Input: dimensioned drawing with shaded views. Units: mm. Origin: part minimum x, y, z. A direction names the side the tool comes from. Round coordinates to 2 decimals unless told otherwise and drop trailing zeros. Order: outer loops, then holes, each group sorted by start corner. A loop starts at its lowest first (then second) coordinate and runs counter-clockwise, first axis right, second up. Notation, with made-up numbers: M 67,60.5 L 122,60.5 A27 ccw 122,82.5 Z; hole C 88,72 d11. An arc over 180 degrees is marked long. Put each result on its own line as item: value. Start each with the question number.
1) Material intervals for probe 1 along Z at (x, y) = (110, 31); probe 2 along X at (y, z) = (25.5, 97.5); probe 3 along Z at (x, y) = (126, 18), sorted ascending. Write a range as [from, to].
2) Section A-A, the plane x = 110. Count the separate pieces of the cut face and the enclosed holes in it, then the cut area to 3 significant figures.
3) First-contact query: P1, Ø10.5, axis at x = 75.5, z = 110, coming from the +Y side; P2, Ø1, axis at y = 14, z = 62.5, coming from the +X side; P3, Ø3, axis at y = 49.5, z = 53, coming from the +X side. Flat tips, straight axial feed; report the tip coordinate or a pass-through.
4) Draft query along Z for the marked faces 1, 2 and 3. Return one class per face: pulls with the +Z half, pulls with the -Z half, needs draft (parallel to the pull), parting line crosses it, or undercut.
5) Section C-C, the plane y = 48. Return loops of the section in (x, z).
6) Access query for the marked faces 4, 5 and 6. Directions: +Z, -Z, +X, -X, +Y, -Y. A direction counts if a zero-diameter tool reaches every point of the face in a straight line with its end or side. Return the directions, or none.
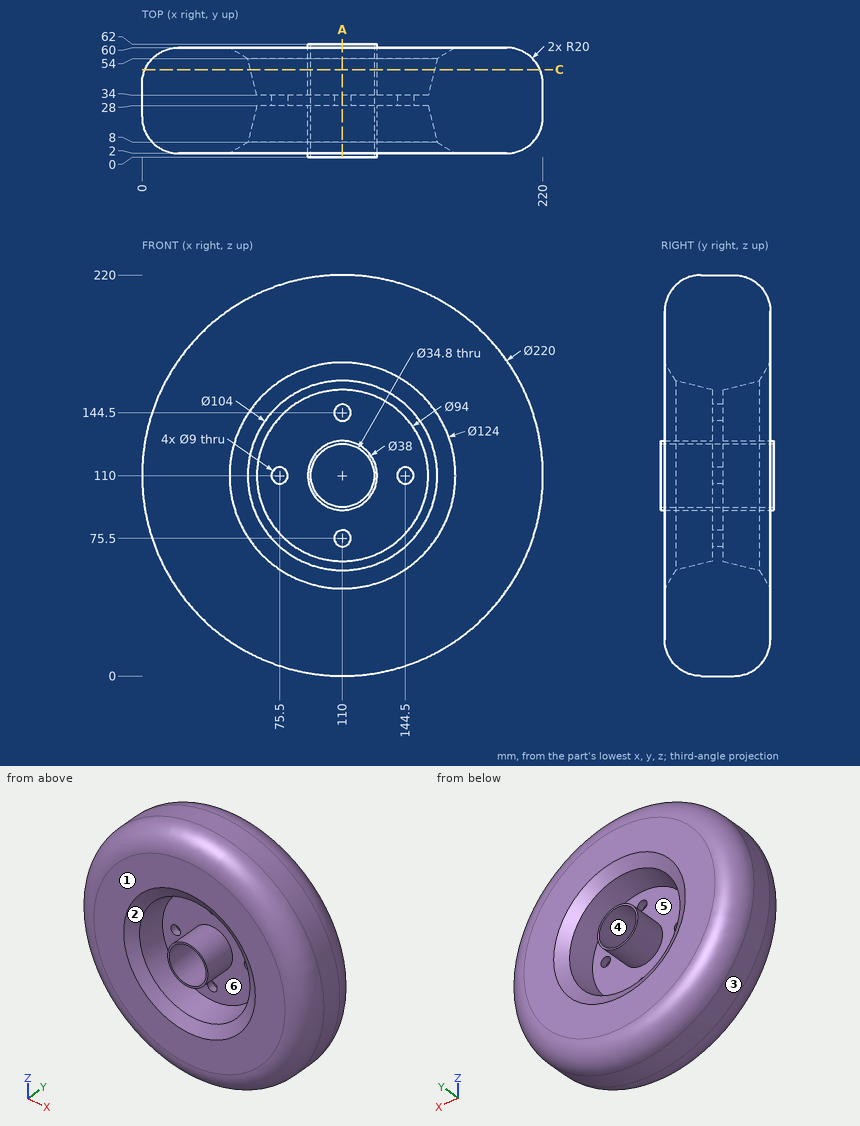
Result sheet:
1. probe 1: z = [0, 71], [80, 92.6], [127.4, 140], [149, 220]
1. probe 2: x = [0.71, 64.04], [95.69, 97.9], [122.1, 124.31], [155.96, 219.29]
1. probe 3: z = [1.58, 63.16], [99.75, 103.16], [116.84, 120.25], [156.84, 218.42]
2. separate pieces: 4
2. enclosed holes: 0
2. area: 6,950 mm2
3. P1: stops at y = 34
3. P2: stops at x = 207.7
3. P3: stops at x = 202.54
4. face 1: needs draft
4. face 2: undercut
4. face 3: parting line crosses it
5. outline: C 110,110 d216.66; C 110,110 d38; hole C 110,110 d101; hole C 110,110 d34.8
6. face 4: +Y, -Y
6. face 5: +Y
6. face 6: -Y
